For this review, take the finished solid that the model builds, in its own axes (mm). A direction names the side the tool comes from. Give positions to 0.01 mm unless a question says otherwise; leave off trailing zeros. Write each loop counter-clockwise with the first axis right and the second up, starting at its lowest first coordinate (ties: lowest second). Pieces come first, ordered by that corner, then holes. Notation, with made-up numbers: M 14,16 L 47,16 A16 ccw 47,30 Z; hole C 3.5,66 d9. An arc over 180 degrees is marked long. Write item = value, one per line.
```python
from build123d import *

# Parameters (mm, degrees)
BOSS_EXTRUDE1_DEPTH = 40
SKETCH2_R           = 60
BOSS_EXTRUDE2_DEPTH = 10
SKETCH3_R           = 58
CUT_EXTRUDE1_DEPTH  = 12
SKETCH5_R           = 68
CUT_EXTRUDE3_DEPTH  = 38


with BuildPart() as part:
    # Sketch1 → Boss-Extrude1 (new body)
    with BuildSketch(Plane(origin=(0, 0, 0), x_dir=(1, 0, 0), z_dir=(0, 1, 0))):
        with BuildLine():
            Line((-30, 70), (30, 70))
            ThreePointArc((30, 70), (58.284271247, 58.284271247), (70, 30))
            Line((70, 30), (70, -30))
            ThreePointArc((70, -30), (58.284271247, -58.284271247), (30, -70))
            Line((30, -70), (-30, -70))
            ThreePointArc((-30, -70), (-58.284271247, -58.284271247), (-70, -30))
            Line((-70, -30), (-70, 30))
            ThreePointArc((-70, 30), (-58.284271247, 58.284271247), (-30, 70))
        make_face()
    extrude(amount=-BOSS_EXTRUDE1_DEPTH)

    # Sketch2 → Boss-Extrude2 (add)
    with BuildSketch(Plane(origin=(0, 0, 0), x_dir=(1, 0, 0), z_dir=(0, 1, 0))):
        with Locations(Location((0, 0, 0), (0, 0, 270))):
            Circle(SKETCH2_R)
    extrude(amount=BOSS_EXTRUDE2_DEPTH)

    # Sketch3 → Cut-Extrude1 (cut)
    with BuildSketch(Plane(origin=(0, 10, 0), x_dir=(1, 0, 0), z_dir=(0, 1, 0))):
        with Locations(Location((0, 0, 0), (0, 0, 270))):
            Circle(SKETCH3_R)
    extrude(amount=-CUT_EXTRUDE1_DEPTH, mode=Mode.SUBTRACT)

    # Sketch5 → Cut-Extrude3 (cut)
    with BuildSketch(Plane.XZ.offset(40)):
        with Locations(Location((0, 0, 0), (0, 0, 270))):
            Circle(SKETCH5_R)
    extrude(amount=-CUT_EXTRUDE3_DEPTH, mode=Mode.SUBTRACT)


solid = part.part
```
1. We need section A-A, the plane x = 0. Write out the cut boundary in (y, z), then the cut area to 3 significant figures.
Responses:
outline = M -40,-70 L 0,-70 L 0,-60 L 10,-60 L 10,-58 L -2,-58 L -2,-68 L -40,-68 Z; M -40,68 L -2,68 L -2,58 L 10,58 L 10,60 L 0,60 L 0,70 L -40,70 Z
area = 240 mm2
2. Insertion check: P1, Ø10, axis at x = 47.5, y = -22.5, coming from the -Z side; P2, Ø2, axis at y = -31, z = -35.5, coming from the +X side; P3, Ø1.5, axis at x = 45, y = -3, coming from the -Z side. Each pin has a flat end and moves straight along its axis. Give the tip position at first contact, or say it passes through.
Responses:
P1 = -68
P2 = 69.75
P3 = -67.38
3. For line 1 along Z through (x, y) = (2, -36.5); line 2 along X through (y, z) = (-25, 0); line 3 along X through (y, z) = (6.25, 0), list the stretches that pass through material, from the lowest coordinate up. Write a range as from..to.
Responses:
line_1 = -70..-67.97, 67.97..70
line_2 = -70..-68, 68..70
line_3 = -60..-58, 58..60
4. The part is to be moulded in two halves that separate along Z. For faces 4 (the face through (-57.972, -19.72, 58.594)), 5 (the face through (31, -2, -50)), 6 (the face through (0, -20, -70)), say which applies: +Z half, -Z half, draft (parallel to the pull), parting line (faces both ways), or undercut.
Responses:
face_4 = +Z half
face_5 = undercut
face_6 = -Z half
5. We need section C-C, the plane y = -14.5. Write out the cut boundary in (x, z), then the cut area to 3 significant figures.
Responses:
outline = M -70,-30 A40 ccw -30,-70 L 30,-70 A40 ccw 70,-30 L 70,30 A40 ccw 30,70 L -30,70 A40 ccw -70,30 Z; hole C 0,0 d136
area = 3,700 mm2
6. Machinability: for faces 1 (the face through (67.42, -21.27, 8.85)), 2 (the face through (-70, -20, 0)), 3 (the face through (2.64, 4.93, -59.94)), which of the approach directions +Z, -Z, +X, -X, +Y, -Y give a long, thin tool a straight path to every point of the face, cutting with its end or side? Answer none if there is none.
Responses:
face_1 = -Y
face_2 = +Z, -Z, -X, +Y, -Y
face_3 = +Y
7. We need section B-B, the plane z = 0. Write out the cut boundary in (x, y).
Responses:
outline = M -70,-40 L -68,-40 L -68,-2 L -58,-2 L -58,10 L -60,10 L -60,0 L -70,0 Z; M 58,-2 L 68,-2 L 68,-40 L 70,-40 L 70,0 L 60,0 L 60,10 L 58,10 Z
